Geometry: final body of the model. Coordinates: model frame, mm. A direction names the side the tool comes from. Give positions to 0.01 mm unless a question says otherwise; leave off trailing zeros. Loops run counter-clockwise (first coordinate to the right, second up) from the corner with the lowest first, then second, coordinate; pieces in that order, holes last. Notation, with made-up numbers: (-13.5, -25.5) - (4.5, -25.5) arc R21 ccw to (4.5, 9.5) - close; hole circle Ø1 at (13.5, 58). An arc over 180 degrees is marked (long way). Use one line per item in the form item = value.
```python
from build123d import *

# Parameters (mm, degrees)
F0_W         = 15
F0_H         = 50
F1_DEPTH     = 16
F3_DEPTH     = 25
F4_T         = -2
F5_R         = 6
F6_R         = 5
F7_DEPTH     = 25
F9_DEPTH     = 4
F10_R        = 5
F11_DEPTH    = 25
F12_T2_ANGLE = 249.8880129875
F12_T4_ANGLE = 220.6883825687
F13_R        = 2
F13_R_2      = 1.25
F14_DEPTH    = 14


# Not quite as in the source:
# - a fillet or chamfer that OpenCascade refuses, or shapes differently, is made with other operations: its cross-section is extruded or revolved along the edge and cut away or added


with BuildPart() as f1:
    # F0 (on Top) → F1 (new body)
    with BuildSketch(Plane.XY):
        with Locations((-7.5, 25)):
            Rectangle(F0_W, F0_H)
    extrude(amount=F1_DEPTH)

    # F2 (on face) → F3 (cut)
    with BuildSketch(Plane.YZ):
        with BuildLine():
            Line((14, 0), (36, 0))
            ThreePointArc((36, 0), (25, 11), (14, 0))
        make_face()
    extrude(amount=-F3_DEPTH, mode=Mode.SUBTRACT)

    # F4
    f4_openings = [f1.faces().sort_by_distance(p)[0] for p in [
        (-7.5, 25, 11),
        (-7.5, 7, 0),
        (-7.5, 43, 0),
    ]]
    offset(amount=F4_T, openings=f4_openings)

    # F5
    f5_edges = [f1.edges().sort_by_distance(p)[0] for p in [
        (0, 0, 8),
        (0, 50, 8),
        (-15, 50, 8),
        (-15, 0, 8),
    ]]
    fillet(f5_edges, radius=F5_R)

    # F6 (on face) → F7 (cut)
    with BuildSketch(Plane.XY.offset(16)):
        with Locations((-7.5, 25)):
            Circle(F6_R)
    extrude(amount=-F7_DEPTH, mode=Mode.SUBTRACT)

    # F8 (on face) → F9 (join)
    with BuildSketch(Plane.XY.offset(16)):
        with BuildLine():
            ThreePointArc((0, 27.7838821814), (-7.5, 33), (-15, 27.7838821814))
            Line((-15, 27.7838821814), (-15, 22.2161178186))
            ThreePointArc((-15, 22.2161178186), (-7.5, 17), (0, 22.2161178186))
            Line((0, 22.2161178186), (0, 27.7838821814))
        make_face()
    extrude(amount=F9_DEPTH)

    # F10 (on face) → F11 (cut)
    with BuildSketch(Plane.XY.offset(20)):
        with Locations((-7.5, 25)):
            Circle(F10_R)
    extrude(amount=-F11_DEPTH, mode=Mode.SUBTRACT)

    # F12: chamfer of 3 on 4 edges, made by hand

    # F12_s1 → F12_t2 (revolve, cut)
    with BuildSketch(Plane(origin=(9.2772397602, 13.2768682197, 0), x_dir=(0, 0, 1), z_dir=(-0.572775629, -0.8197121927, 0))):
        Polygon((20, 15.4672321702), (17, 12.4672321702), (20, 12.4672321702), align=None)
    revolve(axis=Axis((-7.5, 25, 20), (0, 0, 1)), revolution_arc=F12_T2_ANGLE, mode=Mode.SUBTRACT)

    # F12_s3 → F12_t4 (revolve, cut)
    with BuildSketch(Plane(origin=(7.2428078971, 19.5335392611, 0), x_dir=(0, 0, 1), z_dir=(0.3476589265, 0.93762107, 0))):
        Polygon((17, -23.7236311869), (20, -20.7236311869), (20, -23.7236311869), align=None)
    revolve(axis=Axis((-7.5, 25, 20), (0, 0, 1)), revolution_arc=F12_T4_ANGLE, mode=Mode.SUBTRACT)

    # F13 (on face) → F14 (join)
    with BuildSketch(Plane(origin=(0, 0, 14), x_dir=(1, 0, 0), z_dir=(0, 0, -1))):
        with Locations((-7.5, -3)):
            Circle(F13_R)
        with Locations((-7.5, -3)):
            Circle(F13_R_2, mode=Mode.SUBTRACT)
        with Locations((-7.5, -47)):
            Circle(F13_R)
        with Locations((-7.5, -47)):
            Circle(F13_R_2, mode=Mode.SUBTRACT)
    extrude(amount=F14_DEPTH)


solid = f1.part
```
(1) Cut plane A-A (x = -7.5). Return the cut outline in (y, z), plus the area to 3 significant figures.
Solution:
outline = (0, 0) - (2, 0) - (2, 14) - (4.25, 14) - (4.25, 0) - (5, 0) - (5, 14) - (20, 14) - (20, 20) - (17, 17) - (17, 16) - (0, 16) - close; (30, 14) - (45, 14) - (45, 0) - (45.75, 0) - (45.75, 14) - (48, 14) - (48, 0) - (50, 0) - (50, 16) - (33, 16) - (33, 17) - (30, 20) - close
area = 172 mm2
(2) Cut plane B-B (y = 25). Return the cut outline in (x, z).
Solution:
outline = (-15, 11) - (-13, 11) - (-13, 14) - (-12.5, 14) - (-12.5, 20) - (-15, 17.5) - close; (-2.5, 14) - (-2, 14) - (-2, 11) - (0, 11) - (0, 17.5) - (-2.5, 20) - close
(3) Cut plane D-D (y = 12.5). Return the cut outline in (x, z).
Solution:
outline = (-15, 0) - (-13, 0) - (-13, 14) - (-2, 14) - (-2, 0) - (0, 0) - (0, 16) - (-15, 16) - close
(4) Material intervals for L1, parallel to Y at x = -7.5, z = 9.5; L2, parallel to X at y = 9, z = 12; L3, parallel to X at y = 3, z = 7, sorted ascending. Write a range as from..to.
Solution:
L1 = 0..2, 4.25..5, 45..45.75, 48..50
L2 = -15..-13, -2..0
L3 = -14.2..-13, -9.5..-8.75, -6.25..-5.5, -2..-0.8
(5) Pull-direction query (X, two-part tool) for faces 1 (the face through (-4, 2, 7)), 2 (the face through (-8.1, 45.6, 0)), 3 (the face through (-4, 48, 7)), 4 (the face through (-1.804, 48.289, 8.112)); classes: released by +X, released by -X, zero draft, split by the parting line, or undercut.
Solution:
face_1 = undercut
face_2 = zero draft
face_3 = undercut
face_4 = released by +X
(6) Access query for faces 5 (the face through (-13, 25, 12)), 6 (the face through (-5.193, 20.564, 17.042)), 7 (the face through (-7.6, 17, 16.5)). Directions: +Z, -Z, +X, -X, +Y, -Y. A direction counts if a zero-diameter tool reaches every point of the face in a straight line with its end or side. Return the directions, or none.
Solution:
face_5 = -Z
face_6 = +Z, -Z
face_7 = +Z, -Y
(7) Cut plane C-C (z = 10). Return the cut outline in (x, y).
Solution:
outline = (-15, 6) arc R6 ccw to (-9, 0) - (-6, 0) arc R6 ccw to (0, 6) - (0, 20.42) - (-2, 20.42) - (-2, 2) - (-5.77, 2) arc R2 ccw (long way) to (-9.23, 2) - (-13, 2) - (-13, 20.42) - (-15, 20.42) - close; (-15, 29.58) - (-13, 29.58) - (-13, 48) - (-9.23, 48) arc R2 ccw (long way) to (-5.77, 48) - (-2, 48) - (-2, 29.58) - (0, 29.58) - (0, 44) arc R6 ccw to (-6, 50) - (-9, 50) arc R6 ccw to (-15, 44) - close; hole (-8.25, 2) - (-6.75, 2) arc R1.25 ccw (long way) to start; hole (-8.25, 48) arc R1.25 ccw (long way) to (-6.75, 48) - close
(8) Pin query (flat end, axial travel): P1, Ø3, axis at x = -12, z = 5.5, coming from the +Y side; P2, Ø1.1, axis at x = -11, z = 9, coming from the -Y side; P3, Ø4.5, axis at x = -5.5, y = 34.5, coming from the +Z side. Return the tip coordinate at first contact, or that it passes through.
Solution:
P1 = 49.81
P2 = 0.18
P3 = 17.54
